For this review, use the dimensioned drawing (mm, ordinates from the lowest corner) and the shaded views. A direction names the side the tool comes from. Coordinates: 2 decimals unless noted, no trailing zeros. Loops run counter-clockwise (first coordinate to the right, second up) from the corner with the lowest first, then second, coordinate; pieces in that order, holes last. Notation, with made-up numbers: (38, 83.5) - (67, 83.5) arc R26 ccw to (67, 116.5) - close; hole circle Ø6 at (56.5, 18). An arc over 180 degrees is marked (long way). One line per item, written item: value. Start each with the question number.
1. We need section C-C, the plane y = 2.25. Give the boundary of the cut face in (x, z).
2. For the marked faces 1, 2 and 3, list the 3-axis set-ups (+Z, -Z, +X, -X, +Y, -Y) from which the entire face can be reached by the end or side of a thin tool; tool diameter is ignored.
3. We need section D-D, the plane z = 35.5. Give the boundary of the cut face in (x, y), then the cut area to 3 significant figures.
4. We need section A-A, the plane z = 30. Give the boundary of the cut face in (x, y).
5. To check wall thickness, follow line 1 (Z direction, x = 37, y = 0.7); line 2 (X direction, y = 1.45, z = 30); line 3 (X direction, y = 1.9, z = 30). State the ranges of each line that lie inside material, in increasing order.
6. We need section B-B, the plane x = 3. Give the boundary of the cut face in (y, z).
7. Insertion check: P1, Ø8, axis at y = 10, z = 14.5, coming from the -X side; P2, Ø1, axis at x = 31, z = 25, coming from the +Y side; P3, Ø4.5, axis at x = 37.5, z = 17.5, coming from the +Y side; P4, Ø1.5, axis at x = 37, z = 30, coming from the -Y side. Each pin has a flat end and moves straight along its axis. Give the tip position at first contact, or say it passes through.
8. Mouldability with a two-part tool opening along X and no side actions: class the marked faces 4 and 5 as +X half, -X half, draft (parallel to the pull), parting line (faces both ways), or undercut.
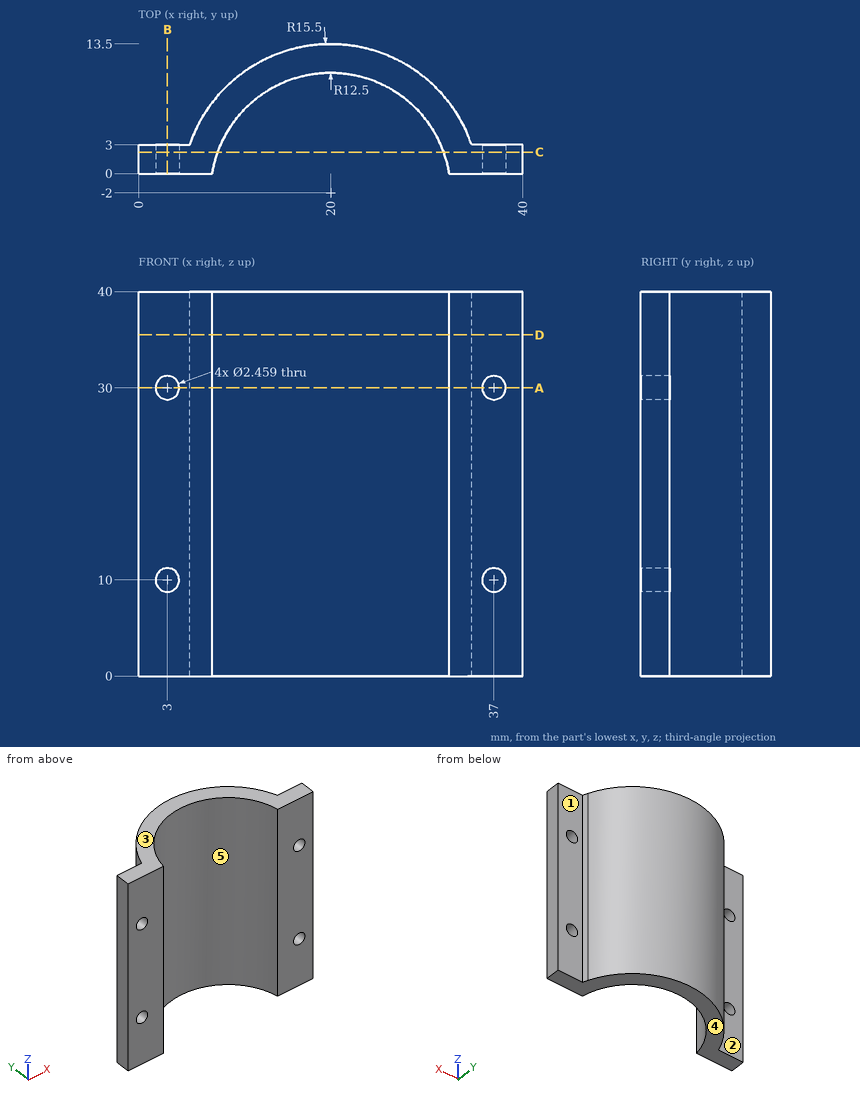
Findings below:
1. outline: (0, 0) - (8.24, 0) - (8.24, 40) - (0, 40) - close; (31.76, 0) - (40, 0) - (40, 40) - (31.76, 40) - close; hole circle Ø2.46 at (3, 10); hole circle Ø2.46 at (3, 30); hole circle Ø2.46 at (37, 10); hole circle Ø2.46 at (37, 30)
2. face 1: +Z, -Z, +X, +Y
2. face 2: +Z, -Z, -X, +Y
2. face 3: +Z, +X, -X, +Y, -Y
3. outline: (0, 0) - (7.66, 0) arc R12.5 cw to (32.34, 0) - (40, 0) - (40, 3) - (34.67, 3) arc R15.5 ccw to (34.29, 4) arc R15.5 ccw to (5.33, 3) - (0, 3) - close
3. area: 149 mm2
4. outline: (0, 0) - (1.77, 0) - (1.77, 3) - (0, 3) - close; (4.23, 0) - (7.66, 0) arc R12.5 cw to (32.34, 0) - (35.77, 0) - (35.77, 3) - (34.67, 3) arc R15.5 ccw to (34.29, 4) arc R15.5 ccw to (5.33, 3) - (4.23, 3) - close; (38.23, 0) - (40, 0) - (40, 3) - (38.23, 3) - close
5. line 1: 0 to 8.77, 11.23 to 28.77, 31.23 to 40
5. line 2: 0 to 1.77, 4.23 to 7.99, 32.01 to 35.77, 38.23 to 40
5. line 3: 0 to 1.77, 4.23 to 8.12, 31.88 to 35.77, 38.23 to 40
6. outline: (0, 0) - (3, 0) - (3, 8.77) - (0, 8.77) - close; (0, 11.23) - (3, 11.23) - (3, 28.77) - (0, 28.77) - close; (0, 31.23) - (3, 31.23) - (3, 40) - (0, 40) - close
7. P1: x = 6.72
7. P2: y = 9.4
7. P3: y = 3
7. P4: through
8. face 4: draft
8. face 5: undercut
